The figure shows three views and two pictorial views of one solid part (mm, origin at its lowest corner). Answer the questions. A direction names the side the tool comes from. Coordinates: 2 decimals unless noted, no trailing zeros. Loops run counter-clockwise (first coordinate to the right, second up) from the corner with the lowest first, then second, coordinate; pieces in that order, holes last. Notation, with made-up numbers: M 87.5,-17 L 143.5,-17 A27 cw 143.5,4 Z; hole C 27.5,61 d7. An arc over 180 degrees is marked long. One line per item, written item: value. Start each with the question number.
1. For the marked faces 1 and 2, determine the directions among +Z, -Z, +X, -X, +Y, -Y from which every point of the face is accessible in a straight line to the end or side of a thin tool.
2. Determine the mould class of the marked faces 3, 4 and 5 for opening direction X: +X half, -X half, draft (parallel to the pull), parting line (faces both ways), or undercut.
3. The part is cut by section D-D (x = 23.75). Write down the section's boundary in (y, z).
4. The part is cut by section B-B (z = 4). Write down the section's boundary in (x, y).
5. The part is cut by section A-A (x = 12). Write down the section's boundary in (y, z), then the cut area to 4 significant figures.
6. Consider probe 1 along Y at (x, z) = (12, 2.1); probe 2 along X at (y, z) = (1.25, 0.6); probe 3 along Y at (x, z) = (13.5, 4.5). Determine where each line is inside the solid, lowest interval first.
7. The part is cut by section C-C (z = 0.5). Write down the section's boundary in (x, y).
8. Flat-ended cylindrical pins translate along their axes: pin 1 (1.5 mm diameter, centred on x = 17.5, y = 3.5, fed in from -Z); pin 2 (2.5 mm diameter, centred on x = 12, y = 4, fed in from +Z). Find the tip coordinate at first contact, or state that the pin passes through.
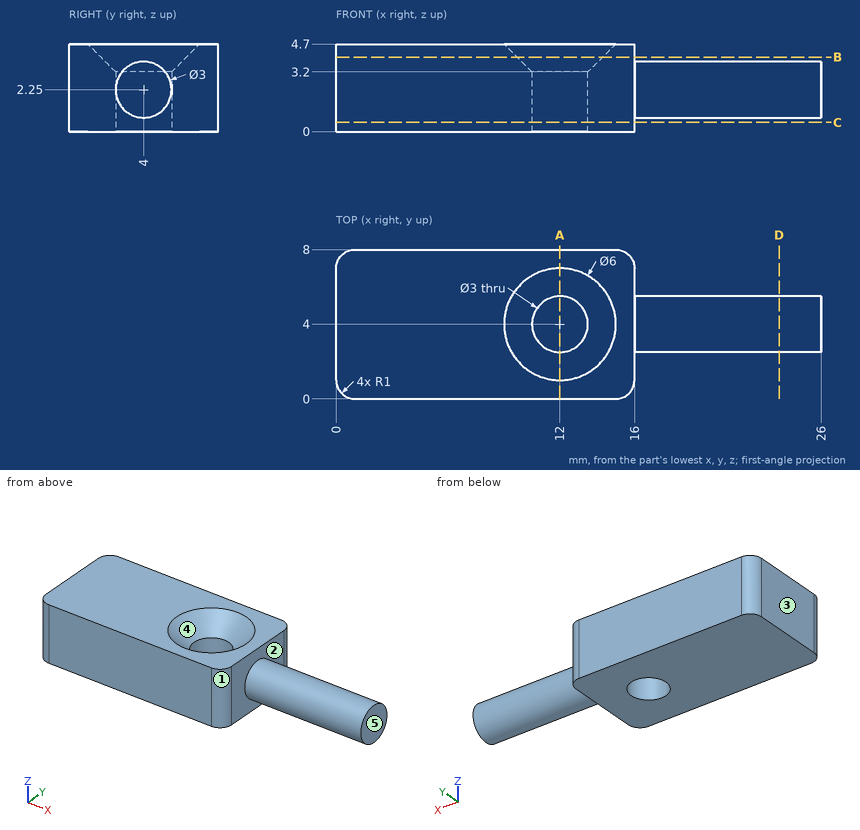
Answer block:
1. face 1: +Z, -Z, +X, -Y
1. face 2: +X
2. face 3: -X half
2. face 4: undercut
2. face 5: +X half
3. outline: C 4,2.25 d3
4. outline: M 0,1 A1 ccw 1,0 L 15,0 A1 ccw 16,1 L 16,7 A1 ccw 15,8 L 1,8 A1 ccw 0,7 Z; hole C 12,4 d4.6
5. outline: M 0,0 L 2.5,0 L 2.5,3.2 L 1,4.7 L 0,4.7 Z; M 5.5,0 L 8,0 L 8,4.7 L 7,4.7 L 5.5,3.2 Z
5. area: 21.25 mm2
6. probe 1: y = 0 to 2.5, 5.5 to 8
6. probe 2: x = 0 to 16
6. probe 3: y = 0 to 1.64, 6.36 to 8
7. outline: M 0,1 A1 ccw 1,0 L 15,0 A1 ccw 16,1 L 16,7 A1 ccw 15,8 L 1,8 A1 ccw 0,7 Z; hole C 12,4 d3
8. pin 1: stops at z = 0.75
8. pin 2: passes through
